from build123d import *

# Parameters (mm, degrees)
F0_W = 15.4980453622
F0_H = 11.90625


with BuildPart() as f1:
    # F0 (on Front) → F1 (revolve)
    with BuildSketch(Plane.XZ):
        with BuildLine():
            Line((-29.3751272816, 20.7111547367), (-30.7169402626, 23.5886819605))
            Line((-30.7169402626, 23.5886819605), (-30.7169402626, 10.0000788365))
            Line((-30.7169402626, 10.0000788365), (-30.7169402626, -1.9061711635))
            Line((-30.7169402626, -1.9061711635), (-10.4812309871, -1.9061711635))
            Line((-10.4812309871, -1.9061711635), (-10.4812309871, 10.0000788365))
            Line((-10.4812309871, 10.0000788365), (-10.4812309871, 23.5886819605))
            Line((-10.4812309871, 23.5886819605), (-11.8230439681, 20.7111547367))
            ThreePointArc((-11.8230439681, 20.7111547367), (-20.5990856249, 14.8884132148), (-29.3751272816, 20.7111547367))
        make_face()
        with Locations((-38.4659629438, 4.0469538365)):
            Rectangle(F0_W, F0_H)
        with Locations((-2.732208306, 4.0469538365)):
            Rectangle(F0_W, F0_H)
    revolve(axis=Axis((-19.7645360604, 0, -1.9061711635), (1, 0, 0)))


solid = f1.part
Geometry check sheet. Reference: the model listing, model coordinates, mm. A direction names the side the tool comes from. Give positions to 0.01 mm unless a question says otherwise; leave off trailing zeros. Write each loop counter-clockwise with the first axis right and the second up, starting at its lowest first coordinate (ties: lowest second). Pieces come first, ordered by that corner, then holes. Notation, with made-up numbers: (73, -38) - (122, -38) arc R36 cw to (122, 1) - close; hole circle Ø10 at (-39, 66). An arc over 180 degrees is marked (long way). Put each result on its own line as item: value.
1. Set-up check for faces 5 (the flat face through (-30.717, 5.3, 9.1)), 6 (the flat face through (-10.481, 5, -13)), 7 (the flat face through (-46.215, 0, -2)): record each of +Z, -Z, +X, -X, +Y, -Y from which the full face is reachable in a straight line by a thin tool's end or side.
Ans:
face 5: -X
face 6: +X
face 7: +Z, -Z, -X, +Y, -Y
2. Sectioned sample at B-B, the plane x = -9. Enter the section's corners in (y, z).
Ans:
outline: circle Ø23.81 at (0, -1.91)
3. Thickness scan on line 1 (X direction, y = -21, z = -9); line 2 (X direction, y = 10.5, z = -8); line 3 (X direction, y = 7.5, z = -21). Record the ranges inside material, lowest first.
Ans:
line 1: x = -30.72 to -29.17, -12.03 to -10.48
line 2: x = -30.72 to -10.48
line 3: x = -30.72 to -28.15, -13.05 to -10.48
4. Go/stop test with flat-tipped pins: pin 1 (8 mm diameter, centred on x = -4, z = 12.5, fed in from -Y); pin 2 (4 mm diameter, centred on x = -14.5, y = -16, fed in from -Z); pin 3 (4 mm diameter, centred on x = -20.5, y = -8.5, fed in from -Z); pin 4 (1 mm diameter, centred on y = 20, z = 16.5, fed in from -X). Record where each tip stops, or that it passes through.
Ans:
pin 1: stops at y = -5.79
pin 2: stops at z = -16.47
pin 3: stops at z = -17.39
pin 4: passes through
5. Sectioned sample at C-C, the plane x = -22.5. Enter the section's corners in (y, z).
Ans:
outline: circle Ø33.97 at (0, -1.91)
6. Draft check along X on faces 1 (the flat face through (5.017, 0, -2)), 2 (the conical face through (-11.758, 22.216, -6.839)), 3 (the cylindrical face through (-38.357, 7.245, -11.355)), 4 (the conical face through (-29.46, -6.85, 19.84)). Enter one of: +X half, -X half, draft (parallel to the pull), parting line (faces both ways), or undercut.
Ans:
face 1: +X half
face 2: undercut
face 3: draft
face 4: undercut
